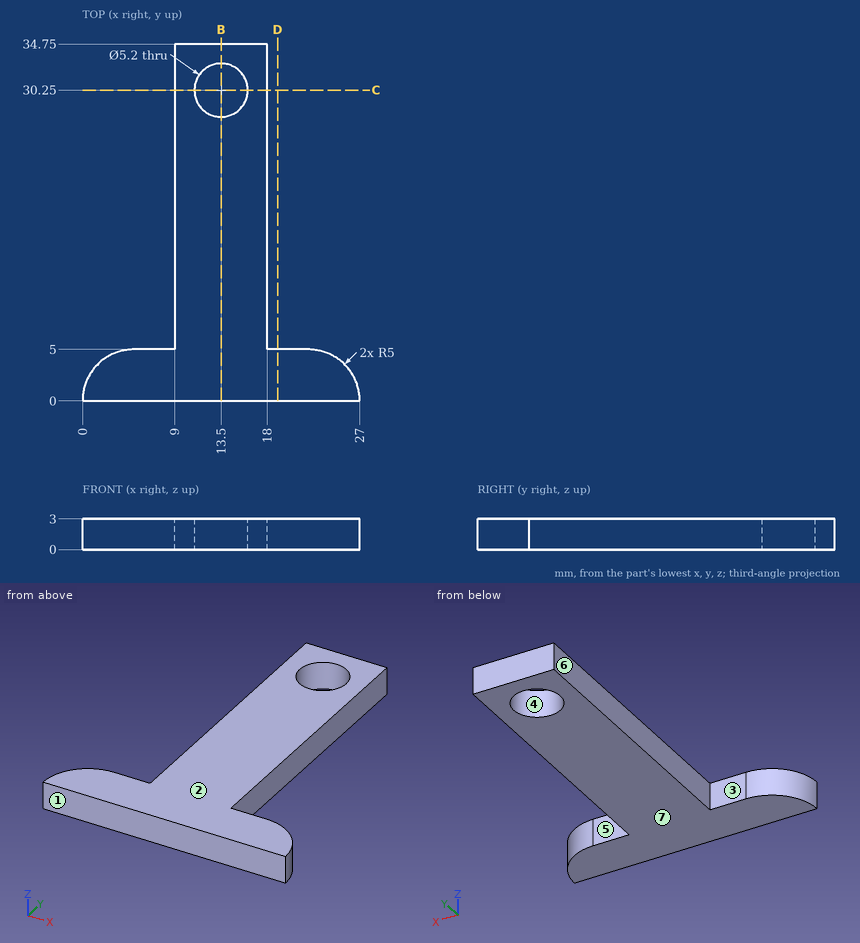
Can you work these out from the drawing? Everything is in mm from the part's minimum corner. A direction names the side the tool comes from. Round coordinates to 2 decimals unless told otherwise and drop trailing zeros. Order: outer loops, then holes, each group sorted by start corner. A loop starts at its lowest first (then second) coordinate and runs counter-clockwise, first axis right, second up. Notation, with made-up numbers: (7.5, 34.25) -> (35.5, 34.25) arc R27 ccw to (35.5, 72.25) -> close; hole circle Ø4 at (18, 71.5). An arc over 180 degrees is marked (long way). Return JSON: item names as keys, results as strings. Group by question number.
1. If we section it at D-D, the plane x = 19: Write out the boundary of the cut face in (y, z).
2. I need wall thicknesses on line 1 (Y direction, x = 13.5, z = 1.1); line 2 (Y direction, x = 26, z = 1.3); line 3 (X direction, y = 16, z = 0.2). Which ranges of each line are inside material? Lowest first, please. Write a range as [from, to].
3. If we section it at C-C, the plane y = 30.25: Write out the boundary of the cut face in (x, z).
4. Which directions (+Z, -Z, +X, -X, +Y, -Y) give clear straight access to the entire face, cutting with the end or side of a thin tool? Please do the marked faces 5, 6 and 7.
5. If we section it at B-B, the plane x = 13.5: Write out the boundary of the cut face in (y, z).
6. We'd pull the mould along Y, two halves only. Please class the marked faces 1, 2, 3 and 4: released by +Y, released by -Y, zero draft, split by the parting line, or undercut.
7. Will these pins go through, and if not, where does the flat tip stop? pin 1 (6 mm diameter, centred on x = 5.5, y = 28, fed in from -Z); pin 2 (1 mm diameter, centred on y = 25.5, z = 1.5, fed in from -X); pin 3 (0.9 mm diameter, centred on y = 18, z = 2, fed in from +X); pin 4 (1.5 mm diameter, centred on x = 20.5, z = 1, fed in from +Y).
Output values:
{
 "1": {"outline": "(0, 0) -> (5, 0) -> (5, 3) -> (0, 3) -> close"},
 "2": {"line 1": "[0, 27.65], [32.85, 34.75]", "line 2": "[0, 3]", "line 3": "[9, 18]"},
 "3": {"outline": "(9, 0) -> (10.9, 0) -> (10.9, 3) -> (9, 3) -> close; (16.1, 0) -> (18, 0) -> (18, 3) -> (16.1, 3) -> close"},
 "4": {"face 5": "+Z, -Z, +X, +Y", "face 6": "+Z, -Z, -X, +Y", "face 7": "-Z, +X, -X, +Y, -Y"},
 "5": {"outline": "(0, 0) -> (27.65, 0) -> (27.65, 3) -> (0, 3) -> close; (32.85, 0) -> (34.75, 0) -> (34.75, 3) -> (32.85, 3) -> close"},
 "6": {"face 1": "released by -Y", "face 2": "zero draft", "face 3": "released by +Y", "face 4": "undercut"},
 "7": {"pin 1": "through", "pin 2": "x = 9", "pin 3": "x = 18", "pin 4": "y = 5"}
}
